The listing builds one solid part. Answer for the finished solid, in the listing's coordinates (mm). A direction names the side the tool comes from. Coordinates: 2 decimals unless noted, no trailing zeros. Order: outer loops, then holes, each group sorted by start corner. A loop starts at its lowest first (then second) coordinate and runs counter-clockwise, first axis right, second up. Notation, with made-up numbers: (31.25, 44.25) -> (49.25, 44.25) arc R20 ccw to (49.25, 48.25) -> close; hole circle Ø4 at (-7, -35.5). An arc over 180 degrees is marked (long way). Answer in a Markdown table with one row per item.
Autodesk Fusion 360 part; units mm, degrees
sketch "Esquisse1" plane through (0, 0, 0) normal (0, 0, 1) x (1, 0, 0)
  line L0 (0, 0) -> (40, 0)
  line L1 (40, 0) -> (40, -10)
  line L2 (40, -10) -> (0, -10)
  line L3 (0, -10) -> (0, 0)
  circle A0 centre (10, -5) radius 3.25
  dimension "d1" = 6.5
extrude "Extrusion1" add sketch "Esquisse1" along normal blind 10
sketch "Esquisse2" plane through (40, 0, 0) normal (1, 0, 0) x (0, 1, 0)
  line L0 (-10, 0) -> (0, 0)
  line L1 (0, 0) -> (0, 10)
  line L2 (0, 10) -> (-10, 10)
  line L3 (-10, 10) -> (-10, 0)
  circle A0 centre (-5, 5) radius 3.1
  dimension "d4" = 6.2
extrude "Extrusion2" cut sketch "Esquisse2" against normal blind 20 contours A0
sketch "Esquisse3" plane through (0, 0, 10) normal (0, 0, 1) x (-1, 0, 0)
  circle A0 centre (-10, 5) radius 3.25
  line L0 (0, 10) -> (-40, 10)
  line L1 (-40, 10) -> (-40, 0)
  line L2 (-40, 0) -> (0, 0)
  line L3 (0, 0) -> (0, 10)
sketch "Esquisse4" plane through (0, 0, 0) normal (0, 0, -1) x (1, 0, 0)
  circle A0 centre (10, 5) radius 3.25
  line L0 (40, 10) -> (0, 10)
  line L1 (0, 10) -> (0, 0)
  line L2 (0, 0) -> (40, 0)
  line L3 (40, 0) -> (40, 10)
sketch "Esquisse5" plane through (0, 0, 10) normal (0, 0, 1) x (-1, 0, 0)
  circle A0 centre (-10, 5) radius 3.25
  dimension "d7" = 6.5
hole "Perçage1" at (10, -5, 10) direction (0, 0, -1) diameter 6.5 depth 73.51 tip angle 118 countersink diameter 10 countersink angle 40
sketch "Esquisse6" plane through (0, 0, 0) normal (0, 0, -1) x (1, 0, 0)
  circle A0 centre (10, 5) radius 3.25
  dimension "d13" = 6.5
hole "Perçage2" at (10, -5, 0) direction (0, 0, 1) diameter 6.5 depth 73.51 tip angle 118 countersink diameter 10 countersink angle 40
(1) Flat-ended cylindrical pins translate along their axes: pin 1 (5.5 mm diameter, centred on y = -5, z = 5, fed in from +X); pin 2 (5 mm diameter, centred on x = 10, y = -5, fed in from +Z). Find the tip coordinate at first contact, or state that the pin passes through.
Check values:
| item | result |
|---|---|
| pin 1 | x = 20 |
| pin 2 | through |
(2) Find the intervals of material crossed by line 1 along Y through (x, z) = (10, 4.9); line 2 along Z through (x, y) = (26.5, -5); line 3 along X through (y, z) = (-6.25, 7.75), in increasing order. Write a range as from..to.
Check values:
| item | result |
|---|---|
| line 1 | -10..-8.25, -1.75..0 |
| line 2 | 0..1.9, 8.1..10 |
| line 3 | 0..6.01, 13.99..20 |
(3) A cutting plane is placed at C-C, the plane z = 6. Determine the outline of the cut face in (x, y), then the cut area to 3 significant figures.
Check values:
| item | result |
|---|---|
| outline | (0, -10) -> (40, -10) -> (40, -7.93) -> (20, -7.93) -> (20, -2.07) -> (40, -2.07) -> (40, 0) -> (0, 0) -> close; hole circle Ø7.09 at (10, -5) |
| area | 243 mm² |
(4) A cutting plane is placed at A-A, the plane y = -5. Determine the outline of the cut face in (x, z).
Check values:
| item | result |
|---|---|
| outline | (0, 0) -> (5, 0) -> (6.75, 4.81) -> (6.75, 5.19) -> (5, 10) -> (0, 10) -> close; (13.25, 4.81) -> (15, 0) -> (40, 0) -> (40, 1.9) -> (20, 1.9) -> (20, 8.1) -> (40, 8.1) -> (40, 10) -> (15, 10) -> (13.25, 5.19) -> close |
(5) For a pull along Z with two mould halves and no side action, classify faces 3 (the flat face through (20, -5, 5)), 4 (the flat face through (20, -10, 5)), 5 (the flat face through (28, -5, 10)) as released by +Z, released by -Z, zero draft, split by the parting line, or undercut.
Check values:
| item | result |
|---|---|
| face 3 | undercut |
| face 4 | zero draft |
| face 5 | released by +Z |
(6) Which of the six approach directions +Z, -Z, +X, -X, +Y, -Y give full straight-line access (tool end or side, diameter ignored) to faces 1 (the cylindrical face through (30.14, -5.672, 1.974)), 2 (the flat face through (40, -2.7, 2.7))?
Check values:
| item | result |
|---|---|
| face 1 | +X |
| face 2 | +Z, -Z, +X, +Y, -Y |
(7) A cutting plane is placed at B-B, the plane z = 4.25. Determine the outline of the cut face in (x, y), then the cut area to 3 significant figures.
Check values:
| item | result |
|---|---|
| outline | (0, -10) -> (40, -10) -> (40, -8.01) -> (20, -8.01) -> (20, -1.99) -> (40, -1.99) -> (40, 0) -> (0, 0) -> close; hole circle Ø6.91 at (10, -5) |
| area | 242 mm² |
(8) A cutting plane is placed at D-D, the plane z = 1.25. Determine the outline of the cut face in (x, y).
Check values:
| item | result |
|---|---|
| outline | (0, -10) -> (40, -10) -> (40, 0) -> (0, 0) -> close; hole circle Ø9.09 at (10, -5) |
